from build123d import *

# Parameters (mm, degrees)
SKETCH_3_R              = 1.175
SKETCH_3_R_2            = 2.5
EXTRUDE_2_DEPTH         = 4
HOLE_WIZARD_1_6_1_6_1_D = 1.6
SKETCH_11_R             = 1.6
CUT_EXTRUDE_1_DEPTH     = 1
SKETCH_12_R             = 3.05
CUT_EXTRUDE_2_DEPTH     = 2


with BuildPart() as part:
    # 草图3 → 凸台-拉伸2 (new body)
    with BuildSketch(Plane(origin=(0, 0, 0), x_dir=(1, 0, 0), z_dir=(0, 1, 0))):
        with BuildLine():
            Line((0, 0), (14.5, 0))
            Line((14.5, 0), (14.5, -6))
            ThreePointArc((14.5, -6), (16.558133666, -11.654675774), (21.769511049, -14.663465909))
            Line((21.769511049, -14.663465909), (27.377359106, -15.652280825))
            ThreePointArc((27.377359106, -15.652280825), (23.392618613, -26.191520443), (12.126111401, -26.331319436))
            Line((12.126111401, -26.331319436), (12.79720876, -22.525337182))
            ThreePointArc((12.79720876, -22.525337182), (11.953704072, -19.377334829), (9, -18))
            Line((9, -18), (0, -18))
            Line((0, -18), (0, 0))
        make_face()
        with Locations(Location((4, -14, 0), (0, 0, 270))):
            Circle(SKETCH_3_R, mode=Mode.SUBTRACT)
        with Locations(Location((4, -8, 0), (0, 0, 270))):
            Circle(SKETCH_3_R, mode=Mode.SUBTRACT)
        with Locations(Location((12.242640687, -3, 0), (0, 0, 270))):
            Circle(SKETCH_3_R, mode=Mode.SUBTRACT)
        with Locations(Location((17.656854249, -18, 0), (0, 0, 270))):
            Circle(SKETCH_3_R_2, mode=Mode.SUBTRACT)
    extrude(amount=EXTRUDE_2_DEPTH)

    # Ø1.6 (1.6) 直径孔1 (through all)
    with Locations(Plane(origin=(0, 4, 0), x_dir=(1, 0, 0), z_dir=(0, 1, 0))):
        with Locations((20.838834765, -21.181980515), (14.474873734, -14.818019485)):
            Hole(HOLE_WIZARD_1_6_1_6_1_D / 2)


with BuildPart() as body_2:
    # 镜向1: mirrored copy
    add(part.part.mirror(Plane(origin=(0, 4, 0), x_dir=(0, 0, 1), z_dir=(1, 0, 0))))

    # 草图11 → 切除-拉伸1 (cut)
    with BuildSketch(Plane(origin=(0, 0, 0), x_dir=(-1, 0, 0), z_dir=(0, -1, 0))):
        with Locations(Location((14.474873734, -14.818019485, 0), (0, 0, 90))):
            Circle(SKETCH_11_R)
        with Locations(Location((20.838834765, -21.181980515, 0), (0, 0, 90))):
            Circle(SKETCH_11_R)
    extrude(amount=-CUT_EXTRUDE_1_DEPTH, mode=Mode.SUBTRACT)

    # 草图12 → 切除-拉伸2 (cut)
    with BuildSketch(Plane(origin=(0, 0, 0), x_dir=(-1, 0, 0), z_dir=(0, -1, 0))):
        with Locations(Location((17.656854249, -18, 0), (0, 0, 90))):
            Circle(SKETCH_12_R)
    extrude(amount=-CUT_EXTRUDE_2_DEPTH, mode=Mode.SUBTRACT)


solid = body_2.part
Can you work these out from the model? Positions are in its coordinate system, mm. A direction names the side the tool comes from. Round coordinates to 2 decimals unless told otherwise and drop trailing zeros. Order: outer loops, then holes, each group sorted by start corner. A loop starts at its lowest first (then second) coordinate and runs counter-clockwise, first axis right, second up. Notation, with made-up numbers: (10.25, 16) - (28.25, 16) arc R34 ccw to (28.25, 46) - close; hole circle Ø6 at (-39, 21). An arc over 180 degrees is marked (long way). Answer in a Markdown table with one row per item.
(1) Suppose I cut it at C-C, the plane x = -16.5. Please give me the cut outline in (y, z), plus the area to 3 significant figures.
From the geometry:
| item | result |
|---|---|
| outline | (0, 11.58) - (4, 11.58) - (4, 15.78) - (2, 15.78) - (2, 15.18) - (0, 15.18) - close; (0, 20.82) - (2, 20.82) - (2, 20.22) - (4, 20.22) - (4, 27.93) - (0, 27.93) - close |
| area | 45.2 mm2 |
(2) Suppose I cut it at D-D, the plane y = 1.4. Please give me the cut outline in (x, z) (3 decimals).
From the geometry:
| item | result |
|---|---|
| outline | (-27.377, 15.652) - (-21.77, 14.663) arc R8.797 cw to (-14.5, 6) - (-14.5, 0) - (0, 0) - (0, 18) - (-9, 18) arc R3.856 cw to (-12.797, 22.525) - (-12.126, 26.331) arc R10 ccw to start; hole circle Ø1.6 at (-20.839, 21.182); hole circle Ø6.1 at (-17.657, 18); hole circle Ø1.6 at (-14.475, 14.818); hole circle Ø2.35 at (-12.243, 3); hole circle Ø2.35 at (-4, 8); hole circle Ø2.35 at (-4, 14) |
(3) Suppose I cut it at B-B, the plane z = 3. Please give me the cut outline in (x, y), plus the area to 3 significant figures.
From the geometry:
| item | result |
|---|---|
| outline | (-14.5, 0) - (-13.42, 0) - (-13.42, 4) - (-14.5, 4) - close; (-11.07, 0) - (0, 0) - (0, 4) - (-11.07, 4) - close |
| area | 48.6 mm2 |
(4) Please list where these lines run through material, in increasing order: L1, parallel to X at y = 1.2, z = 3; L2, parallel to X at y = 1.65, z = 20.5; L3, parallel to Z at x = -8.25, y = 2.55. Write a range as from..to.
From the geometry:
| item | result |
|---|---|
| L1 | x = -14.5..-13.42, -11.07..0 |
| L2 | x = -27.34..-21.26, -20.42..-19.4, -15.91..-12.61 |
| L3 | z = 0..18 |
(5) Which directions (+Z, -Z, +X, -X, +Y, -Y) give clear straight access to the entire face, cutting with the end or side of a thin tool? Please do faces 1 (the face through (-14.5, 2, 3)), 2 (the face through (-13.39, 0.49, 13.64)), 3 (the face through (-5, 2, 18)).
From the geometry:
| item | result |
|---|---|
| face 1 | -Z, -X, +Y, -Y |
| face 2 | -Y |
| face 3 | +Z, +X, +Y, -Y |
(6) Suppose I cut it at A-A, the plane x = -4. Please give me the cut outline in (y, z) (3 decimals).
From the geometry:
| item | result |
|---|---|
| outline | (0, 0) - (4, 0) - (4, 6.825) - (0, 6.825) - close; (0, 9.175) - (4, 9.175) - (4, 12.825) - (0, 12.825) - close; (0, 15.175) - (4, 15.175) - (4, 18) - (0, 18) - close |
(7) If we mould it in two halves opening along Z, with no side actions, what happens to faces 4 (the face through (0, 2, 9)), 5 (the face through (-12.457, 1.972, 24.455)), 6 (the face through (-24.53, 1.97, 15.15))? For each: released by +Z, released by -Z, zero draft, split by the parting line, or undercut.
From the geometry:
| item | result |
|---|---|
| face 4 | zero draft |
| face 5 | undercut |
| face 6 | released by -Z |
(8) For P1, Ø1.8, axis at x = -14.47, z = 14.82, coming from the -Y side; P2, Ø2, axis at y = 2.5, z = 11, coming from the -X side; P3, Ø6, axis at x = -17.66, z = 18, coming from the -Y side, each with a flat end and sliding along its axis, tell me the tip position at first contact or that it passes through.
From the geometry:
| item | result |
|---|---|
| P1 | stops at y = 1 |
| P2 | stops at x = -16.86 |
| P3 | stops at y = 2 |
